CAD build for the part. Positions are in the model's coordinates, mm. A direction names the side the tool comes from. Coordinates: 2 decimals unless noted, no trailing zeros. Order: outer loops, then holes, each group sorted by start corner. A loop starts at its lowest first (then second) coordinate and runs counter-clockwise, first axis right, second up. Notation, with made-up numbers: M 86.25,37.5 L 127.25,37.5 A11 cw 127.25,48.5 Z; hole C 17.25,54 d5. An arc over 180 degrees is marked long. Write item = value, one per line. Start each with the question number.
```python
from build123d import *

# Parameters (mm, degrees)
SKETCH1_W               = 45
SKETCH1_H               = 70
BOSS_EXTRUDE1_DEPTH     = 22
SKETCH2_W               = 20.25
SKETCH2_H               = 9.5
CUT_EXTRUDE1_DEPTH      = 1
CUT_EXTRUDE1_DEPTH_BACK = 46
SKETCH3_R               = 4.2
CUT_EXTRUDE2_DEPTH      = 23
FILLET1_R               = 10
CUT_EXTRUDE3_DEPTH      = 23
FILLET2_R               = 8
FILLET4_R               = 2
CHAMFER1_SIZE           = 0.5
CHAMFER1_SIZE2          = 1.37373871
CHAMFER1_PART_2_SIZE    = 0.5
CHAMFER1_PART_2_SIZE2   = 1.37373871


with BuildPart() as part:
    # Sketch1 → Boss-Extrude1 (new body)
    with BuildSketch(Plane(origin=(0, 0, 0), x_dir=(1, 0, 0), z_dir=(0, 1, 0))):
        Rectangle(SKETCH1_W, SKETCH1_H)
    extrude(amount=BOSS_EXTRUDE1_DEPTH)

    # Sketch2 → Cut-Extrude1 (cut, two sides)
    with BuildSketch(Plane(origin=(22.5, 0, 0), x_dir=(0, 0, -1), z_dir=(1, 0, 0))) as cut_extrude1_sk:
        with Locations((0, 4.75)):
            Rectangle(SKETCH2_W, SKETCH2_H)
    extrude(amount=CUT_EXTRUDE1_DEPTH, mode=Mode.SUBTRACT)
    extrude(cut_extrude1_sk.sketch, amount=-CUT_EXTRUDE1_DEPTH_BACK, mode=Mode.SUBTRACT)

    # Sketch3 → Cut-Extrude2 (cut, through all)
    with BuildSketch(Plane.XZ):
        with Locations((15, 25)):
            Circle(SKETCH3_R)
        with Locations((15, -25)):
            Circle(SKETCH3_R)
        with Locations((-15, -25)):
            Circle(SKETCH3_R)
        with Locations((-15, 25)):
            Circle(SKETCH3_R)
    extrude(amount=-CUT_EXTRUDE2_DEPTH, mode=Mode.SUBTRACT)

    # Fillet1
    fillet1_edges = [part.edges().sort_by_distance(p)[0] for p in [
        (-22.5, 11, -35),
        (22.5, 11, -35),
        (22.5, 11, 35),
        (-22.5, 11, 35),
    ]]
    fillet(fillet1_edges, radius=FILLET1_R)

    # Sketch6 → Cut-Extrude3 (cut, through all)
    with BuildSketch(Plane.XZ):
        with BuildLine():
            Line((12.5, 35), (-12.5, 35))
            ThreePointArc((-12.5, 35), (0, 33.26906369), (12.5, 35))
        make_face()
        with BuildLine():
            Line((12.5, -35), (-12.5, -35))
            ThreePointArc((-12.5, -35), (0, -33.26906369), (12.5, -35))
        make_face()
    extrude(amount=-CUT_EXTRUDE3_DEPTH, mode=Mode.SUBTRACT)

    # Fillet2
    fillet2_edges = [part.edges().sort_by_distance(p)[0] for p in [
        (12.5, 11, 35),
        (-12.5, 11, 35),
        (12.5, 11, -35),
        (-12.5, 11, -35),
    ]]
    fillet(fillet2_edges, radius=FILLET2_R)

    # Fillet4
    fillet4_edges = [part.edges().sort_by_distance(p)[0] for p in [
        (-22.5, 22, 0),
        (22.5, 22, 0),
        (20.63102045, 22, -30.821211768),
        (-20.63102045, 22, 30.821211768),
        (0, 22, 33.26906369),
        (20.63102045, 22, 30.821211768),
        (0, 22, -33.26906369),
        (-20.63102045, 22, -30.821211768),
        (13.473401565, 22, -34.886533438),
        (-13.473401565, 22, -34.886533438),
        (-13.473401565, 22, 34.886533438),
        (13.473401565, 22, 34.886533438),
    ]]
    fillet(fillet4_edges, radius=FILLET4_R)

    # Chamfer1
    chamfer1_edges = [part.edges().sort_by_distance(p)[0] for p in [
        (-19.2, 0, -25),
        (10.8, 0, -25),
    ]]
    chamfer1_side = [part.faces().sort_by_distance(p)[0] for p in [
        (0, 0, -21.437561791),
    ]]
    chamfer(chamfer1_edges, length=CHAMFER1_SIZE, length2=CHAMFER1_SIZE2, reference=chamfer1_side[0])

    # Chamfer1 part 2
    chamfer1_part_2_edges = [part.edges().sort_by_distance(p)[0] for p in [
        (-19.2, 0, 25),
        (10.8, 0, 25),
    ]]
    chamfer1_part_2_side = [part.faces().sort_by_distance(p)[0] for p in [
        (0, 0, 21.437561791),
    ]]
    chamfer(chamfer1_part_2_edges, length=CHAMFER1_PART_2_SIZE, length2=CHAMFER1_PART_2_SIZE2, reference=chamfer1_part_2_side[0])


solid = part.part
```
1. Mould opens along Z. For faces 3 (the flat face through (0, 0, -23)), 4 (the cylindrical face through (-0.16, 9.86, 33.27)), 5 (the cylindrical face through (-20.68, 10.14, -30.75)), 6 (the cylindrical face through (14.453, 11.542, -20.836)) say: released by +Z, released by -Z, zero draft, split by the parting line, or undercut.
2. Flat gauge pins, fed straight in: pin 1 (6.5 mm diameter, centred on x = 15, z = 25, fed in from -Y); pin 2 (3 mm diameter, centred on x = -7.5, y = 3.5, fed in from +Z); pin 3 (6 mm diameter, centred on x = 2.5, y = 10.5, fed in from +Z); pin 4 (6 mm diameter, centred on x = 9, y = 11.5, fed in from -Z). Where does each tip first touch, or does it go through?
3. Slice it at A-A (y = 2.25). Give the number of separate pieces and of enclosed holes in the cut face, plus the area to 3 significant figures.
4. Probe L1, parallel to Z at x = -15, y = 14.25; L2, parallel to Z at x = 17, y = 5 (3 decimals); L3, parallel to X at y = 3.25, z = 28. List the from-to ranges inside material, lowest first.
5. 3-axis set-ups, long thin cutter, end or side, ignore diameter. For faces 1 (the flat face through (0, 5, -10.125)), 2 (the cylindrical face through (-19.196, 11.542, 25.185)): which of +Z, -Z, +X, -X, +Y, -Y reach the whole face in a straight line?
6. Slice it at B-B (z = -7). Write the cut outline in (x, y).
Calculated:
q1.face_3 = zero draft
q1.face_4 = released by +Z
q1.face_5 = released by -Z
q1.face_6 = undercut
q2.pin_1 = through
q2.pin_2 = 34.16
q2.pin_3 = 33.6
q2.pin_4 = -34.81
q3.separate_pieces = 2
q3.enclosed_holes = 4
q3.area = 1,870 mm²
q4.L1 = -34.68 to -29.2, -20.8 to 20.8, 29.2 to 34.68
q4.L2 = -33.93 to -28.693, -21.307 to -10.125, 10.125 to 21.307, 28.693 to 33.93
q4.L3 = -22.04 to -17.94, -12.06 to 12.06, 17.94 to 22.04
q5.face_1 = +X, -X, -Y
q5.face_2 = +Y, -Y
q6.outline = M -22.5,9.5 L 22.5,9.5 L 22.5,20 A2 ccw 20.5,22 L -20.5,22 A2 ccw -22.5,20 Z
